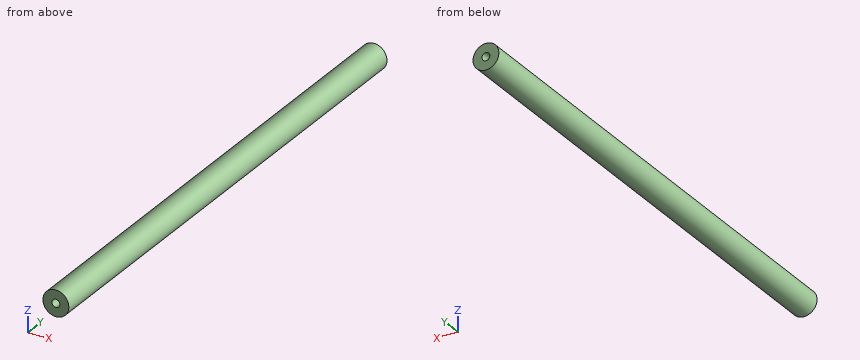
```python
from build123d import *

# Parameters (mm, degrees)
F0_R     = 8
F0_R_2   = 2.455
F1_DEPTH = 320
F4_D     = 4.91
F4_DEPTH = 20
F4_TIP   = 1.4751128197
F5_D     = 4.91
F5_DEPTH = 20
F5_TIP   = 1.4751128197


with BuildPart() as f1:
    # F0 (on Front) → F1 (new body)
    with BuildSketch(Plane.XZ):
        Circle(F0_R)
        Circle(F0_R_2, mode=Mode.SUBTRACT)
        Circle(F0_R_2)
    extrude(amount=F1_DEPTH)

    # F4
    with Locations(Plane.XZ.offset(320)):
        with Locations((0, 0)):
            Hole(F4_D / 2, depth=F4_DEPTH)
            with Locations((0, 0, -(F4_DEPTH + F4_TIP / 2))):  # 118° drill point
                Cone(0, F4_D / 2, F4_TIP, mode=Mode.SUBTRACT)

    # F5
    with Locations(Plane(origin=(0, 0, 0), x_dir=(-1, 0, 0), z_dir=(0, 1, 0))):
        with Locations((0, 0)):
            Hole(F5_D / 2, depth=F5_DEPTH)
            with Locations((0, 0, -(F5_DEPTH + F5_TIP / 2))):  # 118° drill point
                Cone(0, F5_D / 2, F5_TIP, mode=Mode.SUBTRACT)


solid = f1.part
```
Could you check a few things on this model? Use its own coordinates, in mm. Coordinates: 2 decimals unless noted, no trailing zeros. Write each loop counter-clockwise with the first axis right and the second up, starting at its lowest first coordinate (ties: lowest second). Pieces come first, ordered by that corner, then holes. Notation, with made-up numbers: (6.5, -24.75) -> (38.5, -24.75) arc R28 ccw to (38.5, 2.25) -> close; hole circle Ø9 at (11.25, -9.5). An arc over 180 degrees is marked (long way). One line per question, with ' | ' between items. Start each with the question number.
1. Will these pins go through, and if not, where does the flat tip stop? P1, Ø3, axis at x = 3, y = -223, coming from the +Z side; P2, Ø1, axis at x = 4.5, z = 2, coming from the +Y side; P3, Ø3, axis at x = 0, z = 0, coming from the +Y side; P4, Ø3, axis at y = -251.5, z = 3.5, coming from the -X side.
2. If we section it at B-B (x = -5): Please give me the cut outline in (y, z) (3 decimals).
3. If we section it at A-A (y = -171): Please give me the cut outline in (x, z).
4. Please list where these lines run through material, in increasing order: line 1 along Z through (x, y) = (0, -312) (3 decimals); line 2 along X through (y, z) = (-232, 5.5); line 3 along X through (y, z) = (-63, -1).
Return value:
1) P1: stops at z = 7.86 | P2: stops at y = 0 | P3: stops at y = -20.57 | P4: stops at x = -7.75
2) outline: (-320, -6.245) -> (0, -6.245) -> (0, 6.245) -> (-320, 6.245) -> close
3) outline: circle Ø16 at (0, 0)
4) line 1: z = -8 to -2.455, 2.455 to 8 | line 2: x = -5.81 to 5.81 | line 3: x = -7.94 to 7.94
